Can you work these out from the model? Positions are in its coordinate system, mm. A direction names the side the tool comes from. Give positions to 0.01 mm unless a question says otherwise; leave off trailing zeros. Order: outer loops, then holes, each group sorted by start corner. A loop starts at its lowest first (then second) coordinate and runs counter-clockwise, first axis right, second up. Notation, with made-up numbers: (-16, 67.25) - (31, 67.25) arc R20 ccw to (31, 92.25) - close; hole circle Ø9 at (-12, 60). An arc over 180 degrees is marked (long way). Return JSON: item names as keys, results as strings.
```python
from build123d import *

# Parameters (mm, degrees)
SKETCH5_R                = 36.756756757
SKETCH5_R_2              = 20
BOSS_EXTRUDE1_DEPTH      = 3
SKETCH8_R                = 1.75
CUT_EXTRUDE3_DEPTH       = 5
SKETCH27_R               = 1.75
CUT_EXTRUDE9_DEPTH       = 5
SKETCH28_R               = 1.75
CUT_EXTRUDE10_DEPTH      = 10
FILLET1_R                = 3
CIRPATTERN1_COUNT        = 4
FILLET1_OF_CIRPATTERN1_R = 3
SKETCH32_R               = 6
SKETCH32_R_2             = 20
CUT_EXTRUDE11_DEPTH      = 1.7
SKETCH33_R               = 2.7
CUT_EXTRUDE12_DEPTH      = 1.5


with BuildPart() as part:
    # Sketch5 → Boss-Extrude1 (new body)
    with BuildSketch(Plane.XY):
        Circle(SKETCH5_R)
        Circle(SKETCH5_R_2, mode=Mode.SUBTRACT)
    extrude(amount=-BOSS_EXTRUDE1_DEPTH)

    # Sketch8 → Cut-Extrude3 (cut)
    with BuildSketch(Plane.XY):
        with Locations((20.859650045, 20.859650045)):
            Circle(SKETCH8_R)
        with Locations((-20.859650045, 20.859650045)):
            Circle(SKETCH8_R)
        with Locations((-20.859650045, -20.859650045)):
            Circle(SKETCH8_R)
        with Locations((20.859650045, -20.859650045)):
            Circle(SKETCH8_R)
    extrude(amount=-CUT_EXTRUDE3_DEPTH, mode=Mode.SUBTRACT)

    # Sketch27 → Cut-Extrude9 (cut)
    with BuildSketch(Plane.XY):
        with Locations((0, 29.5)):
            Circle(SKETCH27_R)
        with Locations((29.5, 0)):
            Circle(SKETCH27_R)
        with Locations((0, -29.5)):
            Circle(SKETCH27_R)
        with Locations((-29.5, 0)):
            Circle(SKETCH27_R)
    extrude(amount=-CUT_EXTRUDE9_DEPTH, mode=Mode.SUBTRACT)

    # Sketch28 → Cut-Extrude10 (cut)
    with BuildSketch(Plane.XY):
        with BuildLine():
            Line((-3, 36.63412572), (-3, 29.5))
            ThreePointArc((-3, 29.5), (0, 26.5), (3, 29.5))
            Line((3, 29.5), (3, 36.63412572))
            ThreePointArc((3, 36.63412572), (0, 36.756756757), (-3, 36.63412572))
        make_face()
        with Locations((0, 29.5)):
            Circle(SKETCH28_R, mode=Mode.SUBTRACT)
    cut_extrude10 = extrude(amount=-CUT_EXTRUDE10_DEPTH, mode=Mode.SUBTRACT)

    # Fillet1
    fillet1_edges = [part.edges().sort_by_distance(p)[0] for p in [
        (-3, 36.63412572, -1.5),
        (3, 36.63412572, -1.5),
    ]]
    fillet(fillet1_edges, radius=FILLET1_R)

    # CirPattern1: Cut-Extrude10 ×4 about axis
    cirpattern1_axis = Axis((0, 0, 0), (0, 0, 1))
    for i in range(1, CIRPATTERN1_COUNT):
        add(cut_extrude10.rotate(cirpattern1_axis, i * 360 / CIRPATTERN1_COUNT), mode=Mode.SUBTRACT)

    # Fillet1 of CirPattern1
    fillet1_of_cirpattern1_edges = [part.edges().sort_by_distance(p)[0] for p in [
        (-36.63412572, -3, -1.5),
        (-36.63412572, 3, -1.5),
        (3, -36.63412572, -1.5),
        (-3, -36.63412572, -1.5),
        (36.63412572, 3, -1.5),
        (36.63412572, -3, -1.5),
    ]]
    fillet(fillet1_of_cirpattern1_edges, radius=FILLET1_OF_CIRPATTERN1_R)

    # Sketch32 → Cut-Extrude11 (cut)
    with BuildSketch(Plane.XY):
        with Locations((-18.677893379, 7.150964894)):
            Circle(SKETCH32_R)
        Circle(SKETCH32_R_2)
        with Locations((14.366974153, 11.655044131)):
            Circle(SKETCH32_R)
        with Locations((1.745187427, -19.214690235)):
            Circle(SKETCH32_R)
    extrude(amount=-CUT_EXTRUDE11_DEPTH, mode=Mode.SUBTRACT)

    # Sketch33 → Cut-Extrude12 (cut)
    with BuildSketch(Plane(origin=(0, 0, -3), x_dir=(-1, 0, 0), z_dir=(0, 0, -1))):
        with Locations((-20.859650045, 20.859650045)):
            Circle(SKETCH33_R)
        with Locations((20.859650045, 20.859650045)):
            Circle(SKETCH33_R)
        with Locations((20.859650045, -20.859650045)):
            Circle(SKETCH33_R)
        with Locations((-20.859650045, -20.859650045)):
            Circle(SKETCH33_R)
    extrude(amount=-CUT_EXTRUDE12_DEPTH, mode=Mode.SUBTRACT)


solid = part.part
```
1. Suppose I cut it at B-B (z = -2.15). State how many separate pieces and enclosed holes the cut face has, plus the area to 3 significant figures.
Checks:
{"separate pieces": "1", "enclosed holes": "5", "area": "2,640 mm^2"}
2. Suppose I cut it at D-D (y = 14.5). List the corners of the cut face in (x, z) for me.
Checks:
{"outline": "(-33.78, -3) - (-13.77, -3) - (-13.77, 0) - (-33.78, 0) - close; (13.77, -3) - (33.78, -3) - (33.78, 0) - (19.65, 0) - (19.65, -1.7) - (13.77, -1.7) - close"}
3. Suppose I cut it at A-A (y = 4). List the corners of the cut face in (x, z) for me, plus the area to 3 significant figures.
Checks:
{"outline": "(-35.46, -3) - (-19.6, -3) - (-19.6, -1.7) - (-23.78, -1.7) - (-23.78, 0) - (-35.46, 0) - close; (19.6, -3) - (35.46, -3) - (35.46, 0) - (19.6, 0) - close", "area": "88.0 mm^2"}
4. If I drill on L1, parallel to X at y = 0, z = -0.65; L2, parallel to X at y = 12, z = -1.6; L3, parallel to Y at x = 18.5, z = -1.8, over which ranges is the centre line in solid material (lowest first)? Write a range as [from, to].
Checks:
{"L1": "[-26.5, -20], [20, 26.5]", "L2": "[-34.74, -22.21], [20.36, 34.74]", "L3": "[-31.76, -22.17], [-19.55, -7.6], [7.6, 19.55], [22.17, 31.76]"}
5. On a 3-axis mill with a long thin cutter (end or side, diameter ignored), from which of +Z, -Z, +X, -X, +Y, -Y can I reach the whole of each face in a straight line? I mean faces 5 (the face through (17, 14, -1.7)), 6 (the face through (-31, -3, -1)), 7 (the face through (-21, -23, -1.5)). Say none if no direction works.
Checks:
{"face 5": "+Z", "face 6": "+Z, -Z, -X", "face 7": "-Z"}
6. For pin 1 Ø2.5 at (x, y) = (-20.5, 20) entering from -Z; pin 2 Ø1.5 at (x, z) = (30.5, -2) entering from -Y; pin 3 Ø1.5 at (x, z) = (-20.5, -0.5) entering from +Y; pin 4 Ø1.6 at (x, y) = (-20.5, -20.5) entering from -Z, each with a flat end and sliding along its axis, tell me the tip position at first contact or that it passes through.
Checks:
{"pin 1": "z = -1.5", "pin 2": "y = -21.59", "pin 3": "y = 31", "pin 4": "through"}
7. Suppose I cut it at C-C (x = -10). List the corners of the cut face in (y, z) for me, plus the area to 3 significant figures.
Checks:
{"outline": "(-35.37, -3) - (-17.32, -3) - (-17.32, 0) - (-35.37, 0) - close; (17.32, -3) - (35.37, -3) - (35.37, 0) - (17.32, 0) - close", "area": "108 mm^2"}
8. Thinking about a two-plate mould opening in Y: for faces 1 (the face through (-3, -31, -1)), 2 (the face through (21, -23, -1.5)), 3 (the face through (-25.77, 26.21, -1.48)), 4 (the face through (25.77, -26.21, -1.48)), which applies, +Y half, -Y half, draft (parallel to the pull), parting line (faces both ways), or undercut?
Checks:
{"face 1": "draft", "face 2": "undercut", "face 3": "+Y half", "face 4": "-Y half"}
